Here's the drawing with two shaded views (mm, measured from the low corner). I have some questions. Coordinates: 2 decimals unless noted, no trailing zeros. Write each loop counter-clockwise with the first axis right and the second up, starting at its lowest first coordinate (ties: lowest second). Pieces come first, ordered by that corner, then holes. Notation, with made-up numbers: (50, -22) - (74, -22) arc R34 cw to (74, 14) - close; hole circle Ø8 at (-17, -37.75). An arc over 180 degrees is marked (long way). Answer in a Markdown table with one row per item. Add a question column.
Item 1: Imagine slicing it at D-D (z = 12.7). Please give me the cut outline in (x, y) (1 decimal), plus the area to 3 significant figures.
Item 2: Imagine slicing it at B-B (x = 120.65). Please give me the cut outline in (y, z).
Item 3: Imagine slicing it at C-C (x = 48.26). Please give me the cut outline in (y, z) (1 decimal).
Item 4: Imagine slicing it at A-A (z = 106.68). Please give me the cut outline in (x, y).
Item 5: I'm going to push a flat-ended pin straight in: pin 1 (6.5 mm diameter, centred on x = 120.65, z = 50.8, fed in from -Y). Where does the tip first touch, or does it pass through?
Item 6: If I drill on probe 1 along X at (y, z) = (4.35, 12.7) (1 decimal); probe 2 along X at (y, z) = (3, 50.8); probe 3 along Z at (x, y) = (120.65, 5.75), over which ranges is the centre line in solid material (lowest first)? Write a range as from..to.
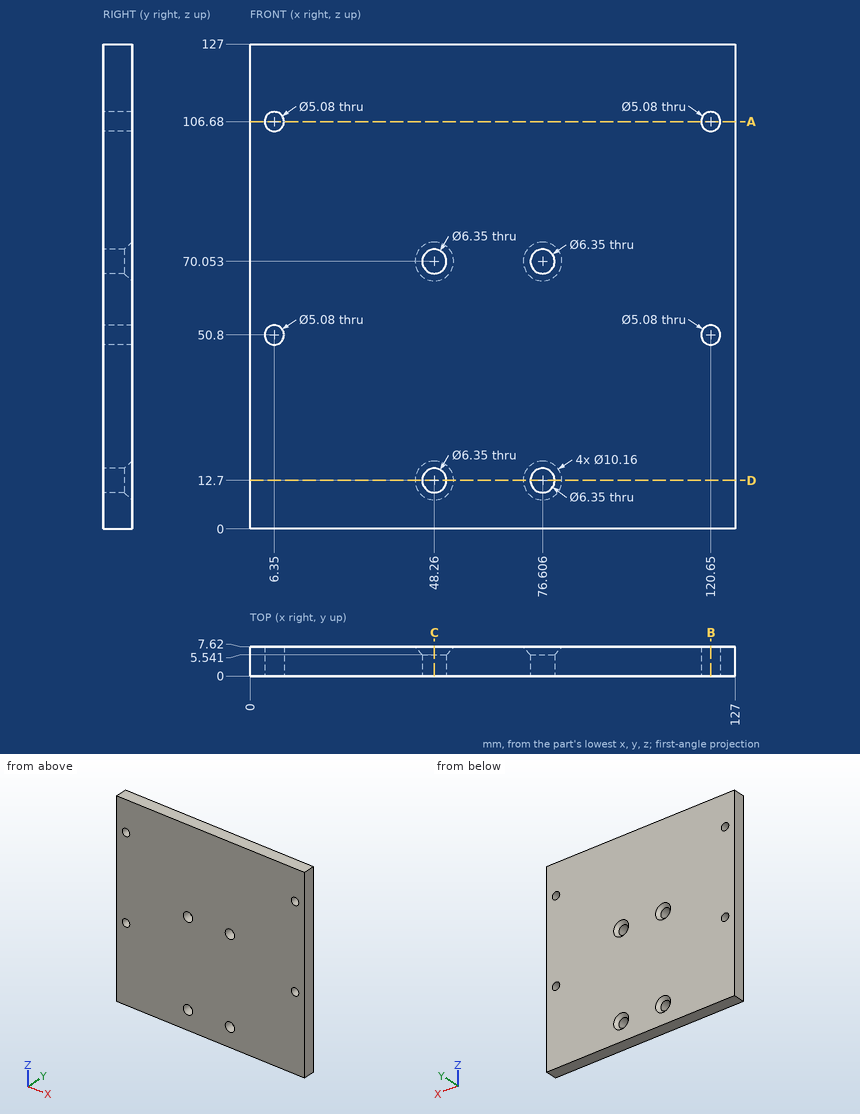
Here are the results:
| question | item | result |
|---|---|---|
| 1 | outline | (0, 0) - (45.1, 0) - (45.1, 5.5) - (43.2, 7.6) - (0, 7.6) - close; (51.4, 0) - (73.4, 0) - (73.4, 5.5) - (71.5, 7.6) - (53.3, 7.6) - (51.4, 5.5) - close; (79.8, 0) - (127, 0) - (127, 7.6) - (81.7, 7.6) - (79.8, 5.5) - close |
| 1 | area | 863 mm2 |
| 2 | outline | (0, 0) - (7.62, 0) - (7.62, 48.26) - (0, 48.26) - close; (0, 53.34) - (7.62, 53.34) - (7.62, 104.14) - (0, 104.14) - close; (0, 109.22) - (7.62, 109.22) - (7.62, 127) - (0, 127) - close |
| 3 | outline | (0, 0) - (7.6, 0) - (7.6, 7.6) - (5.5, 9.5) - (0, 9.5) - close; (0, 15.9) - (5.5, 15.9) - (7.6, 17.8) - (7.6, 65) - (5.5, 66.9) - (0, 66.9) - close; (0, 73.2) - (5.5, 73.2) - (7.6, 75.1) - (7.6, 127) - (0, 127) - close |
| 4 | outline | (0, 0) - (3.81, 0) - (3.81, 7.62) - (0, 7.62) - close; (8.89, 0) - (118.11, 0) - (118.11, 7.62) - (8.89, 7.62) - close; (123.19, 0) - (127, 0) - (127, 7.62) - (123.19, 7.62) - close |
| 5 | pin 1 | stops at y = 0 |
| 6 | probe 1 | x = 0..45.1, 51.4..73.4, 79.8..127 |
| 6 | probe 2 | x = 0..3.81, 8.89..118.11, 123.19..127 |
| 6 | probe 3 | z = 0..48.26, 53.34..104.14, 109.22..127 |
